The listing builds one solid part. Answer for the finished solid, in the listing's coordinates (mm). Give positions to 0.01 mm unless a question says otherwise; leave off trailing zeros. Loops run counter-clockwise (first coordinate to the right, second up) from the corner with the lowest first, then second, coordinate; pieces in that order, holes last. Notation, with made-up numbers: (-1, 42.5) - (17, 42.5) arc R22 cw to (17, 66.5) - close; hole circle Ø8 at (89, -26). An arc over 180 degrees is marked (long way). Answer as CSV lines item,"result". Start each with the question number.
1) A cutting plane is placed at A-A (z = -6.35). Determine the outline of the cut face in (x, y), and give its area (3 significant figures).
2) A cutting plane is placed at B-B (z = 6.35). Determine the outline of the cut face in (x, y).
3) Find the intervals of material crossed by line 1 along X through (y, z) = (0.45, 1.27); line 2 along X through (y, z) = (0.85, -3.81); line 3 along Z through (x, y) = (17.5, 1.25), in increasing order.
```python
from build123d import *

# Parameters (mm, degrees)
SKETCH1_W           = 43.18
SKETCH1_H           = 17.78
SKETCH1_R           = 0.5
BOSS_EXTRUDE1_DEPTH = 1.6
CHAMFER1_SIZE       = 0.3
CHAMFER1_SIZE2      = 0.000523599
CHAMFER2_SIZE       = 0.3
CHAMFER2_SIZE2      = 0.000523599


with BuildPart() as part:
    # Sketch1 → Boss-Extrude1 (new body)
    with BuildSketch(Plane(origin=(0, 0, 0), x_dir=(1, 0, 0), z_dir=(0, 1, 0))):
        Rectangle(SKETCH1_W, SKETCH1_H)
        with Locations(Location((20.32, -6.35, 0), (0, 0, 270))):
            Circle(SKETCH1_R, mode=Mode.SUBTRACT)
        with Locations(Location((-20.32, 3.81, 0), (0, 0, 270))):
            Circle(SKETCH1_R, mode=Mode.SUBTRACT)
        with Locations(Location((-20.32, 1.27, 0), (0, 0, 270))):
            Circle(SKETCH1_R, mode=Mode.SUBTRACT)
        with Locations(Location((-20.32, -1.27, 0), (0, 0, 270))):
            Circle(SKETCH1_R, mode=Mode.SUBTRACT)
        with Locations(Location((-20.32, 6.35, 0), (0, 0, 270))):
            Circle(SKETCH1_R, mode=Mode.SUBTRACT)
        with Locations(Location((-20.32, -3.81, 0), (0, 0, 270))):
            Circle(SKETCH1_R, mode=Mode.SUBTRACT)
        with Locations(Location((-20.32, -6.35, 0), (0, 0, 270))):
            Circle(SKETCH1_R, mode=Mode.SUBTRACT)
        with Locations(Location((17.78, -6.35, 0), (0, 0, 270))):
            Circle(SKETCH1_R, mode=Mode.SUBTRACT)
        with Locations(Location((17.78, -3.81, 0), (0, 0, 270))):
            Circle(SKETCH1_R, mode=Mode.SUBTRACT)
        with Locations(Location((17.78, -1.27, 0), (0, 0, 270))):
            Circle(SKETCH1_R, mode=Mode.SUBTRACT)
        with Locations(Location((20.32, -3.81, 0), (0, 0, 270))):
            Circle(SKETCH1_R, mode=Mode.SUBTRACT)
        with Locations(Location((20.32, -1.27, 0), (0, 0, 270))):
            Circle(SKETCH1_R, mode=Mode.SUBTRACT)
    extrude(amount=BOSS_EXTRUDE1_DEPTH)

    # Chamfer1
    chamfer1_edges = [part.edges().sort_by_distance(p)[0] for p in [
        (20.32, 1.6, 5.85),
        (-20.32, 1.6, -4.31),
        (-20.32, 1.6, -1.77),
        (-20.32, 1.6, 0.77),
        (-20.32, 1.6, 3.31),
        (-20.32, 1.6, 5.85),
        (-20.32, 1.6, -6.85),
        (17.78, 1.6, 5.85),
        (17.78, 1.6, 3.31),
        (17.78, 1.6, 0.77),
        (20.32, 1.6, 3.31),
        (20.32, 1.6, 0.77),
    ]]
    chamfer1_side = [part.faces().sort_by_distance(p)[0] for p in [
        (0.007892141, 1.6, -0.023676424),
    ]]
    chamfer(chamfer1_edges, length=CHAMFER1_SIZE, length2=CHAMFER1_SIZE2, reference=chamfer1_side[0])

    # Chamfer2
    chamfer2_edges = [part.edges().sort_by_distance(p)[0] for p in [
        (20.32, 0, 5.85),
        (-20.32, 0, -4.31),
        (-20.32, 0, -1.77),
        (-20.32, 0, 0.77),
        (-20.32, 0, 3.31),
        (-20.32, 0, 5.85),
        (-20.32, 0, -6.85),
        (17.78, 0, 5.85),
        (17.78, 0, 3.31),
        (17.78, 0, 0.77),
        (20.32, 0, 3.31),
        (20.32, 0, 0.77),
    ]]
    chamfer2_side = [part.faces().sort_by_distance(p)[0] for p in [
        (0.007892141, 0, -0.023676424),
    ]]
    chamfer(chamfer2_edges, length=CHAMFER2_SIZE, length2=CHAMFER2_SIZE2, reference=chamfer2_side[0])


solid = part.part
```
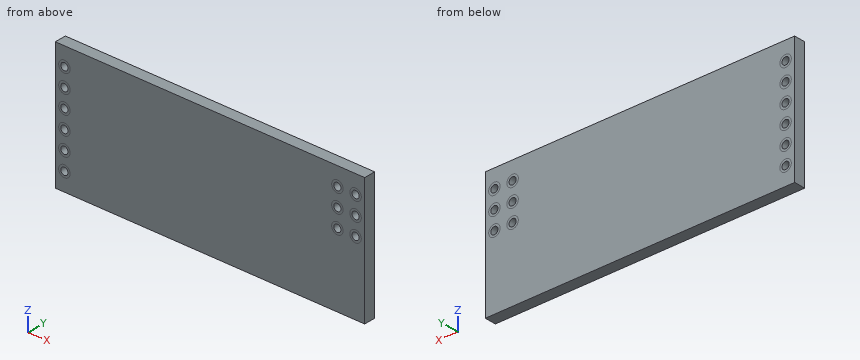
Ans:
1,outline,"(-21.59, 0) - (-21.12, 0) - (-20.82, 0) - (-20.82, 1.6) - (-21.12, 1.6) - (-21.59, 1.6) - close; (-19.82, 0) - (-19.52, 0) - (21.59, 0) - (21.59, 1.6) - (-19.52, 1.6) - (-19.82, 1.6) - close"
1,area,"67.5 mm2"
2,outline,"(-21.59, 0) - (-21.12, 0) - (-20.82, 0) - (-20.82, 1.6) - (-21.12, 1.6) - (-21.59, 1.6) - close; (-19.82, 0) - (-19.52, 0) - (16.98, 0) - (17.28, 0) - (17.28, 1.6) - (16.98, 1.6) - (-19.52, 1.6) - (-19.82, 1.6) - close; (18.28, 0) - (18.58, 0) - (19.52, 0) - (19.82, 0) - (19.82, 1.6) - (19.52, 1.6) - (18.58, 1.6) - (18.28, 1.6) - close; (20.82, 0) - (21.12, 0) - (21.59, 0) - (21.59, 1.6) - (21.12, 1.6) - (20.82, 1.6) - close"
3,line 1,"-21.59 to -20.82, -19.82 to 17.28, 18.28 to 19.82, 20.82 to 21.59"
3,line 2,"-21.59 to -20.82, -19.82 to 21.59"
3,line 3,"-8.89 to 0.86, 1.68 to 3.4, 4.22 to 5.94, 6.76 to 8.89"
